Here's how the part is built. I have some questions about the finished solid (model axes, mm). A direction names the side the tool comes from. Round coordinates to 2 decimals unless told otherwise and drop trailing zeros. Order: outer loops, then holes, each group sorted by start corner. A loop starts at its lowest first (then second) coordinate and runs counter-clockwise, first axis right, second up. Notation, with made-up numbers: M 38,-16 L 62,-16 A24 ccw 62,6 Z; hole C 18,-10 d1. An arc over 180 degrees is marked long. Write each question's results on one line, items separated by ' | '. Start each with the question number.
```python
from build123d import *

# Parameters (mm, degrees)
F0_W     = 5.9
F0_H     = 27
F2_R     = 5.2
F3_DEPTH = 3
F4_R     = 2.6
F5_DEPTH = 25


with BuildPart() as f1:
    # F0 (on Front) → F1 (revolve)
    with BuildSketch(Plane.XZ):
        with Locations((5.399999, 29)):
            Rectangle(F0_W, F0_H)
    revolve(axis=Axis((-4.686111, 0, 0), (-1, 0, 0)))

    # F2 (on face) → F3 (cut)
    with BuildSketch(Plane(origin=(2.449999, 0, 0), x_dir=(0, -1, 0), z_dir=(-1, 0, 0))):
        with Locations((0, 35)):
            Circle(F2_R)
        with Locations((0, -35)):
            Circle(F2_R)
    extrude(amount=-F3_DEPTH, mode=Mode.SUBTRACT)

    # F4 (on face) → F5 (cut)
    with BuildSketch(Plane(origin=(5.449999, 0, 0), x_dir=(0, -1, 0), z_dir=(-1, 0, 0))):
        with Locations((0, -35.2)):
            Circle(F4_R)
        with Locations((0, 35)):
            Circle(F4_R)
    extrude(amount=-F5_DEPTH, mode=Mode.SUBTRACT)


solid = f1.part
```
(1) On a 3-axis mill with a long thin cutter (end or side, diameter ignored), from which of +Z, -Z, +X, -X, +Y, -Y can I reach the whole of each face in a straight line? I mean faces 1 (the cylindrical face through (5.441, 15.368, -2.018)), 2 (the cylindrical face through (3.929, 0.677, -29.844)). Say none if no direction works.
(2) Please list where these lines run through material, in increasing order: line 1 (Y direction, x = 4.65, z = 0); line 2 (X direction, y = -0.5, z = -30); line 3 (Z direction, x = 7.3, y = -14).
(3) I want a section at C-C on y = 9. Write out the boundary of the cut face in (x, z).
(4) I'm going to push flat-ended pins straight in: pin 1 Ø2 at (x, y) = (5, -13.5) entering from -Z; pin 2 Ø2 at (x, z) = (6.5, 19) entering from +Y; pin 3 Ø2 at (x, z) = (7.5, 14) entering from +Y. Where does each tip first touch, or does it pass through?
(5) I want a section at A-A on y = 0. Write out the boundary of the cut face in (x, z), and give its area (3 significant figures).
(6) If we mould it in two halves opening along Z, with no side actions, what happens to faces 3 (the flat face through (5.45, -1.1, -32.6)), 4 (the flat face through (8.35, -18, 1)), 5 (the cylindrical face through (5.441, -25.861, -33.727))? For each: pulls with the +Z half, pulls with the -Z half, needs draft (parallel to the pull), parting line crosses it, or undercut.
(7) I want a section at D-D on z = 35. Write out the boundary of the cut face in (x, y), and give its area (3 significant figures).
(8) I want a section at B-B on z = 0. Write out the boundary of the cut face in (x, y), and give its area (3 significant figures).
Solutions:
1) face 1: +X, -X | face 2: -X
2) line 1: -42.5 to -15.5, 15.5 to 42.5 | line 2: 5.45 to 8.35 | line 3: -40.13 to -6.65, 6.65 to 40.13
3) outline: M 2.45,-41.54 L 8.35,-41.54 L 8.35,-12.62 L 2.45,-12.62 Z; M 2.45,12.62 L 8.35,12.62 L 8.35,41.54 L 2.45,41.54 Z
4) pin 1: z = -40.62 | pin 2: y = 38.5 | pin 3: y = 40.46
5) outline: M 2.45,-42.5 L 8.35,-42.5 L 8.35,-37.8 L 5.45,-37.8 L 5.45,-40.2 L 2.45,-40.2 Z; M 2.45,-29.8 L 5.45,-29.8 L 5.45,-32.6 L 8.35,-32.6 L 8.35,-15.5 L 2.45,-15.5 Z; M 2.45,15.5 L 8.35,15.5 L 8.35,32.4 L 5.45,32.4 L 5.45,29.8 L 2.45,29.8 Z; M 2.45,40.2 L 5.45,40.2 L 5.45,37.6 L 8.35,37.6 L 8.35,42.5 L 2.45,42.5 Z | area: 226 mm^2
6) face 3: undercut | face 4: needs draft | face 5: parting line crosses it
7) outline: M 2.45,-24.11 L 8.35,-24.11 L 8.35,-2.6 L 5.45,-2.6 L 5.45,-5.2 L 2.45,-5.2 Z; M 2.45,5.2 L 5.45,5.2 L 5.45,2.6 L 8.35,2.6 L 8.35,24.11 L 2.45,24.11 Z | area: 238 mm^2
8) outline: M 2.45,-42.5 L 8.35,-42.5 L 8.35,-15.5 L 2.45,-15.5 Z; M 2.45,15.5 L 8.35,15.5 L 8.35,42.5 L 2.45,42.5 Z | area: 319 mm^2
